Autodesk Inventor part; units mm, degrees
ref_plane "YZ Plane" through (0, 0, 0) normal (1, 0, 0) x (0, 1, 0)
ref_plane "XZ Plane" through (0, 0, 0) normal (0, 1, 0) x (-1, 0, 0)
ref_plane "XY Plane" through (0, 0, 0) normal (0, 0, 1) x (1, 0, 0)
sketch "スケッチ1" plane through (0, 0, 0) normal (0, 0, 1) x (1, 0, 0)
  arc A0 (51.7707, 111.0227) -> (0, 122.5) centre (0, 0) ccw
  line L0 (0, 0) -> (0, 122.5) construction
  line L1 (0, 0) -> (122.5, 0) construction
  line L2 (0, 0) -> (51.7707, 111.0227) construction
  arc A1 (48.8124, 104.6785) -> (0, 115.5) centre (0, 0) ccw
  line L3 (0, 122.5) -> (0, 115.5)
  line L4 (51.7707, 111.0227) -> (48.8124, 104.6785)
  dimension "d0" = 122.5
  dimension "d1" = 90
  dimension "d2" = 25
  dimension "d3" = 7
extrude "押し出し1" add sketch "スケッチ1" along normal blind 30
sketch "スケッチ2" plane through (0, 0, 30) normal (0, 0, 1) x (1, 0, 0)
  arc A0 (51.7707, 111.0227) -> (0, 122.5) centre (0, 0) ccw
  arc A1 (30.7995, 114.9452) -> (0, 119) centre (0, 0) ccw construction
  line L0 (0, 122.5) -> (0, 115.5)
  line L1 (48.8124, 104.6785) -> (51.7707, 111.0227)
  point P0 (4.9989, 118.895)
  point P1 (45.7166, 109.8681)
  point P2 (0, 119)
  point P3 (50.2916, 107.8506)
  dimension "d6" = 3.5
  dimension "d7" = 5
  dimension "d8" = 5
hole "穴1" at (4.9989, 118.895, 30) at (45.7166, 109.8681, 30) direction (0, 0, -1) diameter 3.5 depth 8 tip angle 118
properties part number "3D_base-connect"
The listing builds one solid part. Answer for the finished solid, in the listing's coordinates (mm). A direction names the side the tool comes from. Coordinates: 2 decimals unless noted, no trailing zeros. Write each loop counter-clockwise with the first axis right and the second up, starting at its lowest first coordinate (ties: lowest second). Pieces come first, ordered by that corner, then holes. Notation, with made-up numbers: M 9.5,27.25 L 34.5,27.25 A20 ccw 34.5,35.25 Z; hole C 16,5.5 d2. An arc over 180 degrees is marked long. Use a Markdown table: item, result. Add a question column.
1. Section A-A (z = 16.25) is taken. Give the vertices of the cut face in (x, y).
2. Which of the six approach directions +Z, -Z, +X, -X, +Y, -Y give full straight-line access (tool end or side, diameter ignored) to faces 1 (the cylindrical face through (4.922, 120.643, 25.944)), 2 (the flat face through (26, 116, 0))?
3. Section B-B (z = 28) is taken. Count the separate pieces of the cut face and the enclosed holes in it, plus the area to 3 significant figures.
4. For a pull along Y with two mould halves and no side action, classify faces 3 (the flat face through (0, 119, 15)), 4 (the cylindrical face through (24.65, 112.84, 14.79)), 5 (the conical face through (45.81, 109.58, 21.13)) as +Y half, -Y half, draft (parallel to the pull), parting line (faces both ways), or undercut.
5. Section C-C (x = 15) is taken. Give the vertices of the cut face in (y, z), plus the area to 3 significant figures.
6. Straight lines are drawn through the part: line 1 along Y through (x, z) = (3, 9.75); line 2 along Y through (x, z) = (17.5, 17.5); line 3 along Y through (x, z) = (45.5, 22.5). For each, find the intervals that lie inside material, in ascending order. Write a range as [from, to].
7. Given P1, Ø3, axis at x = 45.72, y = 109.87, coming from the +Z side; P2, Ø2, axis at y = 108, z = 11.5, coming from the +X side; P3, Ø3, axis at x = 19, z = 10, coming from the +Y side, each flat-ended and moving along its own axis, determine where each tip first touches the part or whether it passes through.
Data:
| question | item | result |
|---|---|---|
| 1 | outline | M 0,115.5 A115.5 cw 48.81,104.68 L 51.77,111.02 A122.5 ccw 0,122.5 Z |
| 2 | face 1 | +Z |
| 2 | face 2 | -Z, +X, -X, +Y, -Y |
| 3 | separate pieces | 1 |
| 3 | enclosed holes | 2 |
| 3 | area | 344 mm2 |
| 4 | face 3 | draft |
| 4 | face 4 | -Y half |
| 4 | face 5 | undercut |
| 5 | outline | M 114.52,0 L 121.58,0 L 121.58,30 L 114.52,30 Z |
| 5 | area | 212 mm2 |
| 6 | line 1 | y = [115.46, 122.46] |
| 6 | line 2 | y = [114.17, 121.24] |
| 6 | line 3 | y = [106.16, 108.13], [111.6, 113.74] |
| 7 | P1 | stops at z = 21.85 |
| 7 | P2 | stops at x = 50.83 |
| 7 | P3 | stops at y = 121.24 |
